CAD build for the part. Positions are in the model's coordinates, mm. A direction names the side the tool comes from. Round coordinates to 2 decimals unless told otherwise and drop trailing zeros. Loops run counter-clockwise (first coordinate to the right, second up) from the corner with the lowest first, then second, coordinate; pieces in that order, holes last. Notation, with made-up numbers: (67.25, 57.5) - (89.25, 57.5) arc R25 ccw to (89.25, 93.5) - close; hole circle Ø2 at (5.25, -31). An arc over 180 degrees is marked (long way). One line per question, with ' | ' between items.
```python
from build123d import *

# Parameters (mm, degrees)
SKETCH1_R           = 1.5
SKETCH1_R_2         = 3.1
BOSS_EXTRUDE1_DEPTH = 2.2


with BuildPart() as part:
    # Sketch1 → Boss-Extrude1 (new body)
    with BuildSketch(Plane(origin=(0, 0, 0), x_dir=(1, 0, 0), z_dir=(0, 1, 0))):
        Polygon((-145.195425431, -36.865904239), (-153.195425431, -36.865904239), (-153.195425431, -38.865904239), (-161.195425431, -38.865904239), (-161.195425431, -46.687876258), (-154.595425431, -46.687876258), (-154.595425431, -51.187876258), (-161.195425431, -51.187876258), (-161.195425431, -60.865904239), (-152.195425431, -60.865904239), (-152.195425431, -63.065904239), (-161.195425431, -63.065904239), (-161.195425431, -65.065904239), (-137.195425431, -65.065904239), (-137.195425431, -63.065904239), (-146.195425431, -63.065904239), (-146.195425431, -60.865904239), (-137.195425431, -60.865904239), (-137.195425431, -58.865904239), (-137.195425431, -51.865904239), (-138.695425431, -51.865904239), (-138.695425431, -45.865904239), (-137.195425431, -45.865904239), (-137.195425431, -38.865904239), (-145.195425431, -38.865904239), align=None)
        with Locations(Location((-154.852279681, -54.522758488, 0), (0, 0, 270))):
            Circle(SKETCH1_R, mode=Mode.SUBTRACT)
        with Locations(Location((-142.47791101, -55.58341866, 0), (0, 0, 270))):
            Circle(SKETCH1_R, mode=Mode.SUBTRACT)
        with Locations(Location((-149.195425431, -48.865904239, 0), (0, 0, 270))):
            Circle(SKETCH1_R_2, mode=Mode.SUBTRACT)
        with Locations(Location((-155.912939853, -42.148389817, 0), (0, 0, 270))):
            Circle(SKETCH1_R, mode=Mode.SUBTRACT)
        with Locations(Location((-143.538571182, -43.209049989, 0), (0, 0, 270))):
            Circle(SKETCH1_R, mode=Mode.SUBTRACT)
    extrude(amount=BOSS_EXTRUDE1_DEPTH)


solid = part.part
```
(1) Cut at D-D, the plane y = 1.2. State how many separate pieces and enclosed holes the cut face has, then the cut area to 3 significant figures.
Results found:
separate pieces: 1 | enclosed holes: 5 | area: 508 mm²
(2) Cut at C-C, the plane x = -140. Write the cut outline in (y, z), then the cut area to 3 significant figures.
Results found:
outline: (0, 38.87) - (2.2, 38.87) - (2.2, 60.87) - (0, 60.87) - close; (0, 63.07) - (2.2, 63.07) - (2.2, 65.07) - (0, 65.07) - close | area: 52.8 mm²
(3) Tool access for faces 1 (the face through (-157, 1, 38.866)), 2 (the face through (-141, 1, 38.866)), 3 (the face through (-142, 1, 63.066)), 4 (the face through (-161.195, 1, 43)), 5 (the face through (-152.195, 1, 62)): list every direction of +Z, -Z, +X, -X, +Y, -Y with a clear straight run to the whole face (end or side of a thin tool).
Results found:
face 1: -Z, -X, +Y, -Y | face 2: -Z, +X, +Y, -Y | face 3: +X, +Y, -Y | face 4: +Z, -Z, -X, +Y, -Y | face 5: -X, +Y, -Y
(4) Two-plate mould, pull along X, no slides. Class faces 6 (the face through (-149, 1, 36.866)), 7 (the face through (-154.595, 1, 49)), 8 (the face through (-142.05, 1.08, 43.01)): released by +X, released by -X, zero draft, split by the parting line, or undercut.
Results found:
face 6: zero draft | face 7: released by -X | face 8: undercut
(5) Probe L1, parallel to X at y = 0.9, z = 55.5; L2, parallel to X at y = 1.55, z = 42.75; L3, parallel to Z at x = -153, y = 0.4. List the from-to ranges inside material, lowest first.
Results found:
L1: x = -161.2 to -155.99, -153.71 to -143.98, -140.98 to -137.2 | L2: x = -161.2 to -157.29, -154.54 to -144.97, -142.11 to -137.2 | L3: z = 36.87 to 60.87, 63.07 to 65.07
(6) Cut at A-A, the plane x = -158.75. Write the cut outline in (y, z), then the cut area to 3 significant figures.
Results found:
outline: (0, 38.87) - (2.2, 38.87) - (2.2, 46.69) - (0, 46.69) - close; (0, 51.19) - (2.2, 51.19) - (2.2, 60.87) - (0, 60.87) - close; (0, 63.07) - (2.2, 63.07) - (2.2, 65.07) - (0, 65.07) - close | area: 42.9 mm²
(7) Cut at B-B, the plane z = 43. Write the cut outline in (x, y).
Results found:
outline: (-161.2, 0) - (-157.15, 0) - (-157.15, 2.2) - (-161.2, 2.2) - close; (-154.68, 0) - (-145.02, 0) - (-145.02, 2.2) - (-154.68, 2.2) - close; (-142.05, 0) - (-137.2, 0) - (-137.2, 2.2) - (-142.05, 2.2) - close
(8) Drop flat-ended pins along their axis: P1, Ø0.7, axis at x = -157, y = 0.5, coming from the -Z side; P2, Ø1.1, axis at y = 1, z = 61.5, coming from the -X side; P3, Ø2.5, axis at x = -142.48, z = 55.58, coming from the +Y side; P4, Ø1.1, axis at y = 1.5, z = 49, coming from the -X side. Give the stop position or say it passes through.
Results found:
P1: stops at z = 38.87 | P2: stops at x = -152.2 | P3: passes through | P4: stops at x = -154.6
